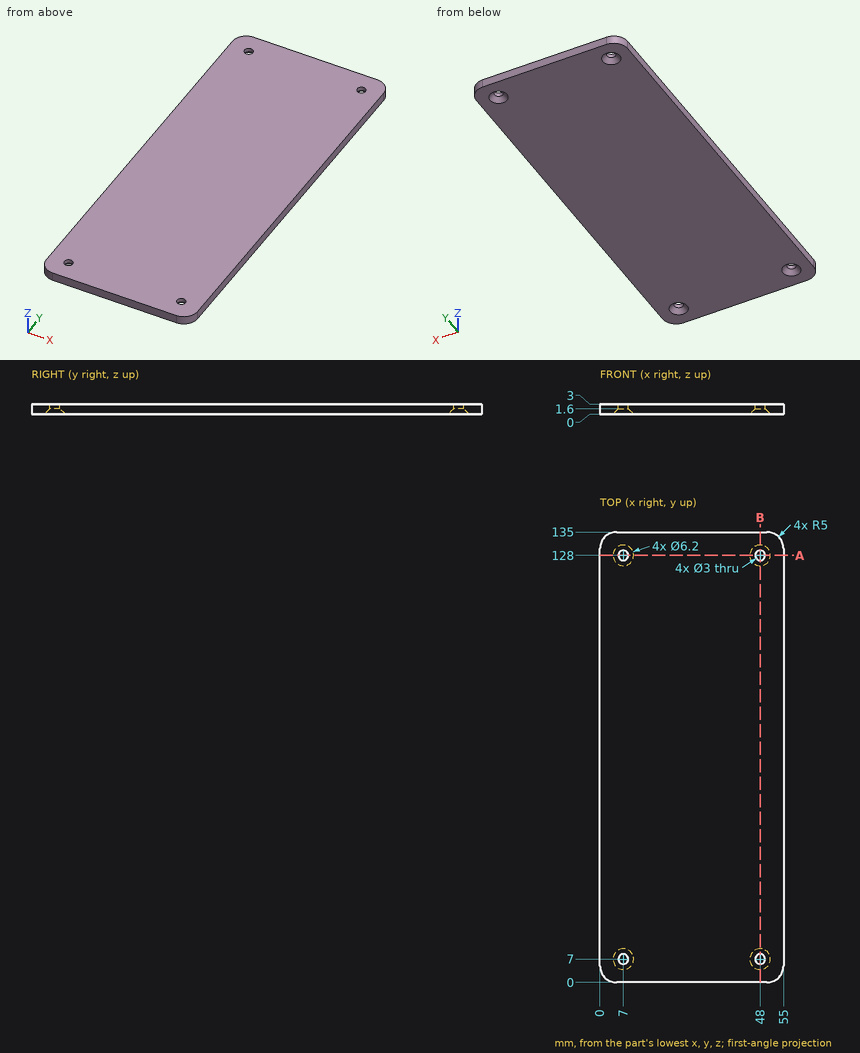
The figure shows three views and two pictorial views of one solid part (mm, origin at its lowest corner). Answer the questions. Give positions to 0.01 mm unless a question says otherwise; leave off trailing zeros. Loops run counter-clockwise (first coordinate to the right, second up) from the corner with the lowest first, then second, coordinate; pieces in that order, holes last. Notation, with made-up numbers: (-20.75, 15.5) - (1.25, 15.5) arc R28 ccw to (1.25, 46.5) - close; hole circle Ø9 at (6, 48.5). An arc over 180 degrees is marked (long way). Answer in a Markdown table with one row per item.
(1) Consider L1, parallel to Y at x = 48, z = 2.55; L2, parallel to X at y = 7, z = 2.4; L3, parallel to X at y = 127, z = 1.75. Determine where each line is inside the solid, lowest interval first. Write a range as [from, to].
Results list:
| item | result |
|---|---|
| L1 | y = [0, 5.5], [8.5, 126.5], [129.5, 135] |
| L2 | x = [0, 5.5], [8.5, 46.5], [49.5, 55] |
| L3 | x = [0, 5.88], [8.12, 46.88], [49.12, 55] |
(2) Section A-A (y = 128) is taken. Give the vertices of the cut face in (x, z).
Results list:
| item | result |
|---|---|
| outline | (0, 0) - (3.9, 0) - (5.5, 1.6) - (5.5, 3) - (0, 3) - close; (8.5, 1.6) - (10.1, 0) - (44.9, 0) - (46.5, 1.6) - (46.5, 3) - (8.5, 3) - close; (49.5, 1.6) - (51.1, 0) - (55, 0) - (55, 3) - (49.5, 3) - close |
(3) Flat-ended cylindrical pins translate along their axes: pin 1 Ø1.8 at (x, y) = (7, 128) entering from +Z; pin 2 Ø3.5 at (x, y) = (48, 128) entering from -Z. Find the tip coordinate at first contact, or state that the pin passes through.
Results list:
| item | result |
|---|---|
| pin 1 | passes through |
| pin 2 | stops at z = 1.35 |
(4) Section B-B (x = 48) is taken. Give the vertices of the cut face in (y, z).
Results list:
| item | result |
|---|---|
| outline | (0, 0) - (3.9, 0) - (5.5, 1.6) - (5.5, 3) - (0, 3) - close; (8.5, 1.6) - (10.1, 0) - (124.9, 0) - (126.5, 1.6) - (126.5, 3) - (8.5, 3) - close; (129.5, 1.6) - (131.1, 0) - (135, 0) - (135, 3) - (129.5, 3) - close |
